```python
from build123d import *

# Parameters (mm, degrees)
SKETCH_1_R      = 3
EXTRUDE_1_DEPTH = 4
EXTRUDE_2_DEPTH = 14
SKETCH_4_R      = 1
EXTRUDE_3_DEPTH = 1.5
SKETCH_5_R      = 5
EXTRUDE_4_DEPTH = 2
EXTRUDE_START   = 2
SKETCH_6_R      = 5
EXTRUDE_5_DEPTH = 2
FILLET_1_R      = 4


with BuildPart() as part:
    # 草图1 → 凸台-拉伸1 (new body)
    with BuildSketch(Plane.XY):
        Circle(SKETCH_1_R)
    extrude(amount=EXTRUDE_1_DEPTH)

    # 草图2 → 凸台-拉伸2 (add)
    with BuildSketch(Plane.XY):
        Polygon((1, 0), (1, 2), (-1, 2), (-1, -2), (1, -2), align=None)
    extrude(amount=EXTRUDE_2_DEPTH)

    # 草图4 → 凸台-拉伸3 (add, symmetric)
    with BuildSketch(Plane(origin=(0, 0, 0), x_dir=(0, 0, -1), z_dir=(1, 0, 0))):
        with Locations(Location((-10, 0, 0), (0, 0, 90))):
            Circle(SKETCH_4_R)
    extrude(amount=EXTRUDE_3_DEPTH, both=True)

    # 草图5 → 凸台-拉伸4 (add)
    with BuildSketch(Plane.ZY.offset(1.5)):
        with Locations((10, 0)):
            Circle(SKETCH_5_R)
    extrude(amount=EXTRUDE_4_DEPTH)

    # 草图6 → 凸台-拉伸5 (add)
    with BuildSketch(Plane(origin=(1.5, 0, 0), x_dir=(0, 0, -1), z_dir=(1, 0, 0)).offset(EXTRUDE_START)):
        with Locations(Location((-10, 0, 0), (0, 0, 180))):
            Circle(SKETCH_6_R)
    extrude(amount=-EXTRUDE_5_DEPTH)

    # 圆角1
    fillet_1_edges = [part.edges().sort_by_distance(p)[0] for p in [
        (0, 2, 14),
    ]]
    fillet(fillet_1_edges, radius=FILLET_1_R - 0.0001)  # a hair under: the kernel refuses the full size


solid = part.part
```
Input: part model. Units: mm. Frame: model coordinates. A direction names the side the tool comes from. Give positions to 0.01 mm unless a question says otherwise; leave off trailing zeros. Order: outer loops, then holes, each group sorted by start corner. A loop starts at its lowest first (then second) coordinate and runs counter-clockwise, first axis right, second up.
1. Material intervals for L1, parallel to X at y = 1.25, z = 8.75; L2, parallel to X at y = -2.25, z = 12.25; L3, parallel to Y at x = 0, z = 4.5, sorted ascending.
Derived:
L1: x = -3.5 to -1.5, -1 to 1, 1.5 to 3.5
L2: x = -3.5 to -1.5, 1.5 to 3.5
L3: y = -2 to 2
2. Section B-B on y = 1.75. Return the cut outline in (x, z).
Derived:
outline: (-3.5, 5.32) - (-1.5, 5.32) - (-1.5, 14.68) - (-3.5, 14.68) - close; (-2.44, 0) - (2.44, 0) - (2.44, 4) - (1, 4) - (1, 11.39) - (-1, 11.39) - (-1, 4) - (-2.44, 4) - close; (1.5, 5.32) - (3.5, 5.32) - (3.5, 14.68) - (1.5, 14.68) - close
3. Pin query (flat end, axial travel): pin 1 (3 mm diameter, centred on x = -2.5, y = 4, fed in from -Z); pin 2 (0.6 mm diameter, centred on x = -0.5, z = 9, fed in from -Y); pin 3 (1.5 mm diameter, centred on x = -0.5, y = -3, fed in from +Z). Return the tip coordinate at first contact, or that it passes through.
Derived:
pin 1: stops at z = 5.67
pin 2: stops at y = -2
pin 3: stops at z = 4
4. Section A-A on z = 5.5. Return the cut outline in (x, y).
Derived:
outline: (-3.5, -2.18) - (-1.5, -2.18) - (-1.5, 2.18) - (-3.5, 2.18) - close; (-1, -2) - (1, -2) - (1, 2) - (-1, 2) - close; (1.5, -2.18) - (3.5, -2.18) - (3.5, 2.18) - (1.5, 2.18) - close
5. Mould query, pull axis Z, two halves, no side actions, for faces 4 (the cylindrical face through (1.25, -0.13, 10.99)), 5 (the cylindrical face through (-0.014, 0.859, 12.797)), 6 (the flat face through (3.5, 0, 10)). Classes: released by +Z, released by -Z, zero draft, split by the parting line, or undercut.
Derived:
face 4: undercut
face 5: released by +Z
face 6: zero draft
6. Reachability of faces 1 (the flat face through (0, 2, 7)), 2 (the cylindrical face through (-1.25, -0.13, 10.99)), 3 (the cylindrical face through (-3, 0, 2)) from +Z, -Z, +X, -X, +Y, -Y: full face, straight path, thin tool, end or side. Return the list, or none.
Derived:
face 1: +Z, +Y
face 2: none
face 3: -Z
7. Section D-D on y = 3.5. Return the cut outline in (x, z), and give its area (3 significant figures).
Derived:
outline: (-3.5, 6.43) - (-1.5, 6.43) - (-1.5, 13.57) - (-3.5, 13.57) - close; (1.5, 6.43) - (3.5, 6.43) - (3.5, 13.57) - (1.5, 13.57) - close
area: 28.6 mm2
